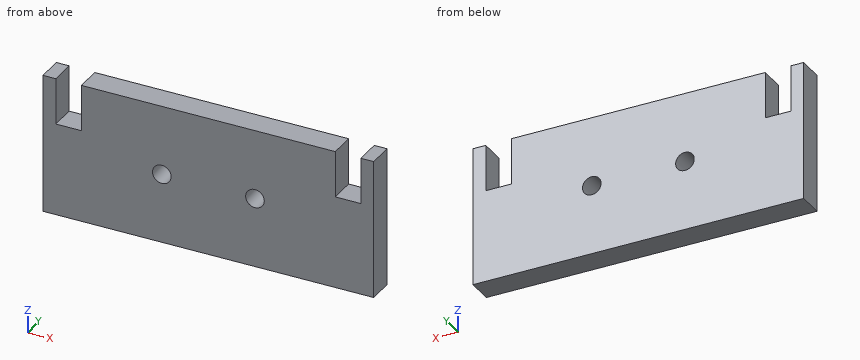
Autodesk Inventor part; units mm, degrees
ref_plane "YZ Plane" through (0, 0, 0) normal (1, 0, 0) x (0, 1, 0)
ref_plane "XZ Plane" through (0, 0, 0) normal (0, 1, 0) x (-1, 0, 0)
ref_plane "XY Plane" through (0, 0, 0) normal (0, 0, 1) x (1, 0, 0)
sketch "Sketch1" plane through (0, 0, 0) normal (0, 1, 0) x (-1, 0, 0)
  line L0 (35.5, -15) -> (-35.5, -15)
  line L1 (-35.5, -15) -> (-35.5, 15)
  line L2 (-35.5, 15) -> (35.5, 15)
  line L3 (35.5, 15) -> (35.5, -15)
  line L4 (35.5, -15) -> (-35.5, 15) construction
  line L5 (-35.5, -15) -> (35.5, 15) construction
  point P0 (0, 0)
  dimension "d0" = 71
  dimension "d5" = 30
extrude "Extrusion1" add sketch "Sketch1" along normal blind 5.5
sketch "Sketch3" plane through (0, 5.5, 0) normal (0, 1, 0) x (1, 0, 0)
  line L0 (-35.5, -15) -> (35.5, -15)
  line L1 (0, 22.4425) -> (0, -29.6547)
  line L2 (-27.25, -15) -> (-32.75, -15)
  line L3 (-32.75, -15) -> (-32.75, -5)
  line L4 (-32.75, -5) -> (-27.25, -5)
  line L5 (-27.25, -5) -> (-27.25, -15)
  line L6 (-30, -0.7186) -> (-30, -17.2123)
  line L7 (27.25, -15) -> (32.75, -15)
  line L8 (32.75, -15) -> (32.75, -5)
  line L9 (32.75, -5) -> (27.25, -5)
  line L10 (27.25, -5) -> (27.25, -15)
  point P0 (0, 0)
  dimension "d6" = 5.5
  dimension "d7" = 10
  dimension "d8" = 30
extrude "Extrusion2" cut sketch "Sketch3" against normal through all
sketch "Sketch4" plane through (0, 5.5, 0) normal (0, 1, 0) x (1, 0, 0)
  line L0 (-27.25, -5) -> (-27.25, -15)
  line L1 (-27.25, -15) -> (27.25, -15)
  line L2 (27.25, -15) -> (27.25, -5)
  line L3 (27.25, -5) -> (32.75, -5)
  line L4 (32.75, -5) -> (32.75, -15)
  line L5 (32.75, -15) -> (35.5, -15)
  line L6 (35.5, -15) -> (35.5, 15)
  line L7 (35.5, 15) -> (-35.5, 15)
  line L8 (-35.5, 15) -> (-35.5, -15)
  line L9 (-35.5, -15) -> (-32.75, -15)
  line L10 (-32.75, -15) -> (-32.75, -5)
  line L11 (-32.75, -5) -> (-27.25, -5)
  point P0 (0, 0)
sketch "Sketch5" plane through (0, 0, 0) normal (0, -1, 0) x (1, 0, 0)
  line L0 (-49.7, 0) -> (49.7, 0)
  line L1 (0, -21) -> (0, 21)
  circle A0 centre (-10, 0) radius 2
  circle A1 centre (10, 0) radius 2
  point P0 (0, 0)
  dimension "d11" = 4
  dimension "d12" = 20
extrude "Extrusion3" cut sketch "Sketch5" against normal through all
equation "\"d1\" = Wt"
equation "\"d6\" = Wt"
properties part number "ex_holder_stopper" material "Wood (Birch)"
Source: CAD feature listing. Evaluate the final solid. Frame: model axes, mm. Coordinates: 2 decimals unless noted, no trailing zeros. Order: outer loops, then holes, each group sorted by start corner. A loop starts at its lowest first (then second) coordinate and runs counter-clockwise, first axis right, second up. Notation, with made-up numbers: M 5.25,7 L 35.25,7 A26 cw 35.25,29 Z; hole C 10.5,-32 d1. An arc over 180 degrees is marked long. Write each question's results on one line, items separated by ' | '. Start each with the question number.
Item 1: Cut plane C-C (z = 0). Return loops of the section in (x, y).
Item 2: Line query: probe 1 along X at (y, z) = (3.9, 9.5); probe 2 along X at (y, z) = (2.7, 0); probe 3 along Z at (x, y) = (10, 4). Output: solid intervals per line, ascending.
Item 3: Cut plane B-B (y = 3.4). Return loops of the section in (x, z), and give its area (3 significant figures).
Item 4: Cut plane A-A (x = -10). Return loops of the section in (y, z).
Item 5: Cut plane D-D (z = 9.25). Return loops of the section in (x, y), and give its area (3 significant figures).
Checked values:
1) outline: M -35.5,0 L -12,0 L -12,5.5 L -35.5,5.5 Z; M -8,0 L 8,0 L 8,5.5 L -8,5.5 Z; M 12,0 L 35.5,0 L 35.5,5.5 L 12,5.5 Z
2) probe 1: x = -35.5 to -32.75, -27.25 to 27.25, 32.75 to 35.5 | probe 2: x = -35.5 to -12, -8 to 8, 12 to 35.5 | probe 3: z = -15 to -2, 2 to 15
3) outline: M -35.5,-15 L 35.5,-15 L 35.5,15 L 32.75,15 L 32.75,5 L 27.25,5 L 27.25,15 L -27.25,15 L -27.25,5 L -32.75,5 L -32.75,15 L -35.5,15 Z; hole C -10,0 d4; hole C 10,0 d4 | area: 1,990 mm2
4) outline: M 0,-15 L 5.5,-15 L 5.5,-2 L 0,-2 Z; M 0,2 L 5.5,2 L 5.5,15 L 0,15 Z
5) outline: M -35.5,0 L -32.75,0 L -32.75,5.5 L -35.5,5.5 Z; M -27.25,0 L 27.25,0 L 27.25,5.5 L -27.25,5.5 Z; M 32.75,0 L 35.5,0 L 35.5,5.5 L 32.75,5.5 Z | area: 330 mm2
